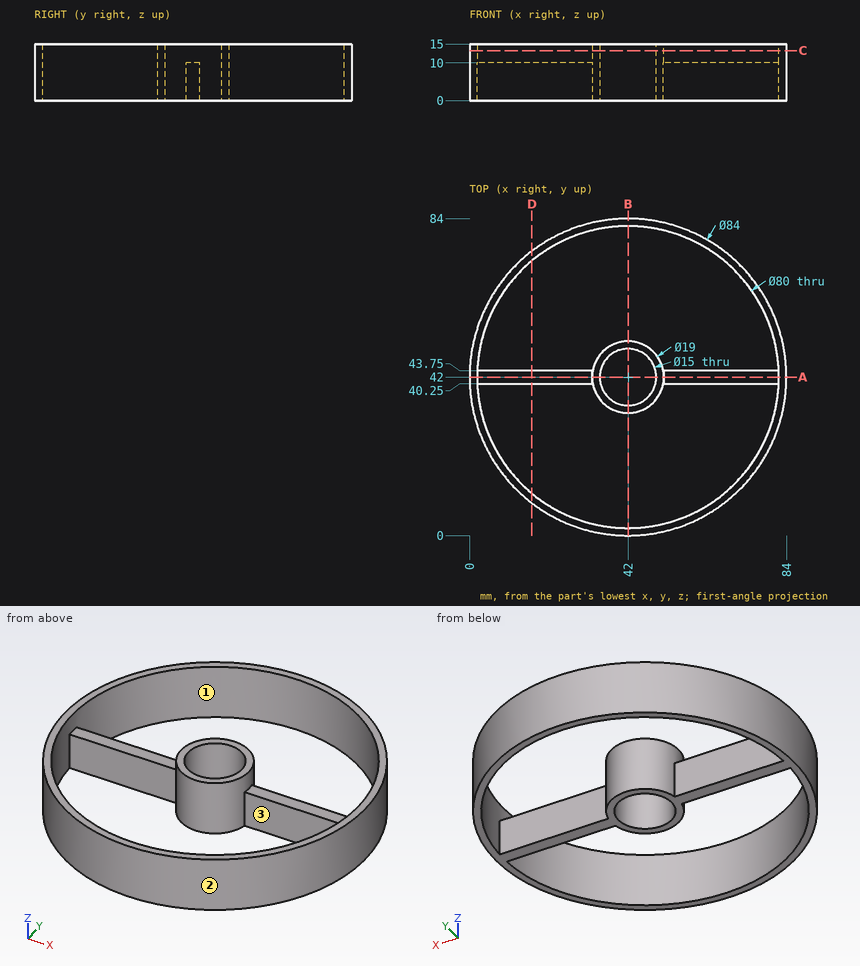
Here's the drawing with two shaded views (mm, measured from the low corner). I have some questions. Coordinates: 2 decimals unless noted, no trailing zeros. Order: outer loops, then holes, each group sorted by start corner. A loop starts at its lowest first (then second) coordinate and runs counter-clockwise, first axis right, second up.
Q1. Will these pins go through, and if not, where does the flat tip stop? pin 1 (19.5 mm diameter, centred on x = 42, y = 42, fed in from -Z); pin 2 (8 mm diameter, centred on x = 66, z = 5.5, fed in from +Y); pin 3 (2 mm diameter, centred on y = 32, z = 13.5, fed in from -X); pin 4 (4 mm diameter, centred on x = 19, z = 2, fed in from +Y).
Q2. Suppose I cut it at A-A on y = 42. Please give me the cut outline in (x, z).
Q3. Thinking about a two-plate mould opening in Y: for the marked faces 1, 2 and 3, which applies, released by +Y, released by -Y, zero draft, split by the parting line, or undercut?
Q4. Suppose I cut it at D-D on x = 16.5. Please give me the cut outline in (y, z), and give its area (3 significant figures).
Q5. Suppose I cut it at C-C on z = 13.25. Please give me the cut outline in (x, y), and give its area (3 significant figures).
Q6. Please list where these lines run through material, in increasing order: L1, parallel to Y at x = 42, z = 8.5; L2, parallel to Y at x = 37.5, z = 8.75; L3, parallel to Y at x = 76.5, z = 7.75.
Q7. Suppose I cut it at B-B on x = 42. Please give me the cut outline in (y, z), and give its area (3 significant figures).
Answer:
1. pin 1: stops at z = 0
1. pin 2: stops at y = 78.93
1. pin 3: stops at x = 0.98
1. pin 4: stops at y = 78.37
2. outline: (0, 0) - (34.5, 0) - (34.5, 15) - (32.5, 15) - (32.5, 10) - (2, 10) - (2, 15) - (0, 15) - close; (49.5, 0) - (84, 0) - (84, 15) - (82, 15) - (82, 10) - (51.5, 10) - (51.5, 15) - (49.5, 15) - close
3. face 1: undercut
3. face 2: split by the parting line
3. face 3: undercut
4. outline: (8.63, 0) - (11.18, 0) - (11.18, 15) - (8.63, 15) - close; (40.25, 0) - (43.75, 0) - (43.75, 10) - (40.25, 10) - close; (72.82, 0) - (75.37, 0) - (75.37, 15) - (72.82, 15) - close
4. area: 112 mm2
5. outline: circle Ø84 at (42, 42); circle Ø19 at (42, 42); hole circle Ø80 at (42, 42); hole circle Ø15 at (42, 42)
5. area: 622 mm2
6. L1: y = 0 to 2, 32.5 to 34.5, 49.5 to 51.5, 82 to 84
6. L2: y = 0.24 to 2.25, 33.63 to 36, 48 to 50.37, 81.75 to 83.76
6. L3: y = 18.05 to 21.76, 40.25 to 43.75, 62.24 to 65.95
7. outline: (0, 0) - (2, 0) - (2, 15) - (0, 15) - close; (32.5, 0) - (34.5, 0) - (34.5, 15) - (32.5, 15) - close; (49.5, 0) - (51.5, 0) - (51.5, 15) - (49.5, 15) - close; (82, 0) - (84, 0) - (84, 15) - (82, 15) - close
7. area: 120 mm2
